Geometry: final body of the model. Coordinates: model frame, mm. A direction names the side the tool comes from. Round coordinates to 2 decimals unless told otherwise and drop trailing zeros. Write each loop counter-clockwise with the first axis right and the second up, starting at its lowest first coordinate (ties: lowest second). Pieces come first, ordered by that corner, then holes.
from build123d import *

# Parameters (mm, degrees)
SKETCH1_W               = 304.8
SKETCH1_H               = 171.45
BOSS_EXTRUDE1_DEPTH     = 19.05
SKETCH2_W               = 19.05
SKETCH2_H               = 19.05
BOSS_EXTRUDE2_DEPTH     = 19.05
SKETCH3_W               = 19.05
SKETCH3_H               = 19.05
CUT_EXTRUDE1_DEPTH      = 367.928913415
CUT_EXTRUDE2_DEPTH      = 367.928913415
CUT_EXTRUDE2_DEPTH_BACK = 367.928913415
CUT_EXTRUDE3_DEPTH      = 367.928913415
CUT_EXTRUDE3_DEPTH_BACK = 367.928913415
CUT_EXTRUDE4_DEPTH      = 367.928913415
SKETCH9_W               = 241.3
SKETCH9_H               = 171.45
BOSS_EXTRUDE3_DEPTH     = 19.05


with BuildPart() as part:
    # Sketch1 → Boss-Extrude1 (new body)
    with BuildSketch(Plane(origin=(0, 0, 0), x_dir=(1, 0, 0), z_dir=(0, 1, 0))):
        with Locations((-152.4, 85.725)):
            Rectangle(SKETCH1_W, SKETCH1_H)
    extrude(amount=BOSS_EXTRUDE1_DEPTH)

    # Mirror1: part across plane


with BuildPart() as part_1:
    add(part.part)
    add(part.part.mirror(Plane(origin=(0, 19.05, 0), x_dir=(0, 0, 1), z_dir=(-1, 0, 0))))

    # Sketch2 → Boss-Extrude2 (add)
    with BuildSketch(Plane(origin=(0, 19.05, 0), x_dir=(1, 0, 0), z_dir=(0, 1, 0))):
        with Locations((-314.325, 28.575)):
            Rectangle(SKETCH2_W, SKETCH2_H)
        with Locations((-314.325, 104.775)):
            Rectangle(SKETCH2_W, SKETCH2_H)
        with Locations((314.325, 142.875)):
            Rectangle(SKETCH2_W, SKETCH2_H)
        with Locations((314.325, 66.675)):
            Rectangle(SKETCH2_W, SKETCH2_H)
    extrude(amount=-BOSS_EXTRUDE2_DEPTH)

    # Sketch3 → Cut-Extrude1 (cut, symmetric)
    with BuildSketch(Plane(origin=(0, 19.05, 0), x_dir=(1, 0, 0), z_dir=(0, 1, 0))):
        with Locations((-104.775, 9.525)):
            Rectangle(SKETCH3_W, SKETCH3_H)
        with Locations((-104.775, 161.925)):
            Rectangle(SKETCH3_W, SKETCH3_H)
    cut_extrude1 = extrude(amount=CUT_EXTRUDE1_DEPTH, both=True, mode=Mode.SUBTRACT)

    # Mirror2: Cut-Extrude1 across plane
    add(cut_extrude1.mirror(Plane(origin=(0, 0, 0), x_dir=(0, 0, 1), z_dir=(1, 0, 0))), mode=Mode.SUBTRACT)

    # Sketch5 → Cut-Extrude2 (cut, two sides: drawn at the far end of the back side and taken through both)
    with BuildSketch(Plane(origin=(0, 19.05, 0), x_dir=(1, 0, 0), z_dir=(0, 1, 0)).offset(-CUT_EXTRUDE2_DEPTH_BACK)):
        with BuildLine():
            Line((9.525, 131.490128061), (9.525, 141.559871939))
            ThreePointArc((9.525, 141.559871939), (9.525, 146.05), (5.034871939, 146.05))
            Line((5.034871939, 146.05), (-5.034871939, 146.05))
            ThreePointArc((-5.034871939, 146.05), (-9.525, 146.05), (-9.525, 141.559871939))
            Line((-9.525, 141.559871939), (-9.525, 131.490128061))
            ThreePointArc((-9.525, 131.490128061), (-9.525, 127), (-5.034871939, 127))
            Line((-5.034871939, 127), (5.034871939, 127))
            ThreePointArc((5.034871939, 127), (9.525, 127), (9.525, 131.490128061))
        make_face()
        with BuildLine():
            Line((9.525, 80.690128061), (9.525, 90.759871939))
            ThreePointArc((9.525, 90.759871939), (9.525, 95.25), (5.034871939, 95.25))
            Line((5.034871939, 95.25), (-5.034871939, 95.25))
            ThreePointArc((-5.034871939, 95.25), (-9.525, 95.25), (-9.525, 90.759871939))
            Line((-9.525, 90.759871939), (-9.525, 80.690128061))
            ThreePointArc((-9.525, 80.690128061), (-9.525, 76.2), (-5.034871939, 76.2))
            Line((-5.034871939, 76.2), (5.034871939, 76.2))
            ThreePointArc((5.034871939, 76.2), (9.525, 76.2), (9.525, 80.690128061))
        make_face()
        with BuildLine():
            Line((9.525, 29.890128061), (9.525, 39.959871939))
            ThreePointArc((9.525, 39.959871939), (9.525, 44.45), (5.034871939, 44.45))
            Line((5.034871939, 44.45), (-5.034871939, 44.45))
            ThreePointArc((-5.034871939, 44.45), (-9.525, 44.45), (-9.525, 39.959871939))
            Line((-9.525, 39.959871939), (-9.525, 29.890128061))
            ThreePointArc((-9.525, 29.890128061), (-9.525, 25.4), (-5.034871939, 25.4))
            Line((-5.034871939, 25.4), (5.034871939, 25.4))
            ThreePointArc((5.034871939, 25.4), (9.525, 25.4), (9.525, 29.890128061))
        make_face()
    extrude(amount=CUT_EXTRUDE2_DEPTH + CUT_EXTRUDE2_DEPTH_BACK, mode=Mode.SUBTRACT)

    # Sketch6 → Cut-Extrude3 (cut, two sides: drawn at the far end of the back side and taken through both)
    with BuildSketch(Plane(origin=(0, 19.05, 0), x_dir=(1, 0, 0), z_dir=(0, 1, 0)).offset(-CUT_EXTRUDE3_DEPTH_BACK)):
        with BuildLine():
            Line((-114.3, 166.959871939), (-114.3, 156.890128061))
            ThreePointArc((-114.3, 156.890128061), (-114.3, 152.4), (-109.809871939, 152.4))
            Line((-109.809871939, 152.4), (-99.740128061, 152.4))
            ThreePointArc((-99.740128061, 152.4), (-95.25, 152.4), (-95.25, 156.890128061))
            Line((-95.25, 156.890128061), (-95.25, 166.959871939))
            Line((-95.25, 166.959871939), (-114.3, 166.959871939))
        make_face()
        with BuildLine():
            ThreePointArc((114.3, 156.890128061), (114.3, 152.4), (109.809871939, 152.4))
            Line((109.809871939, 152.4), (99.740128061, 152.4))
            ThreePointArc((99.740128061, 152.4), (95.25, 152.4), (95.25, 156.890128061))
            Line((95.25, 156.890128061), (95.25, 166.959871939))
            Line((95.25, 166.959871939), (114.3, 166.959871939))
            Line((114.3, 166.959871939), (114.3, 156.890128061))
        make_face()
        with BuildLine():
            ThreePointArc((95.25, 14.559871939), (95.25, 19.05), (99.740128061, 19.05))
            Line((99.740128061, 19.05), (109.809871939, 19.05))
            ThreePointArc((109.809871939, 19.05), (114.3, 19.05), (114.3, 14.559871939))
            Line((114.3, 14.559871939), (114.3, 4.490128061))
            Line((114.3, 4.490128061), (95.25, 4.490128061))
            Line((95.25, 4.490128061), (95.25, 14.559871939))
        make_face()
        with BuildLine():
            Line((-95.25, 4.490128061), (-95.25, 14.559871939))
            ThreePointArc((-95.25, 14.559871939), (-95.25, 19.05), (-99.740128061, 19.05))
            Line((-99.740128061, 19.05), (-109.809871939, 19.05))
            ThreePointArc((-109.809871939, 19.05), (-114.3, 19.05), (-114.3, 14.559871939))
            Line((-114.3, 14.559871939), (-114.3, 4.490128061))
            Line((-114.3, 4.490128061), (-95.25, 4.490128061))
        make_face()
    extrude(amount=CUT_EXTRUDE3_DEPTH + CUT_EXTRUDE3_DEPTH_BACK, mode=Mode.SUBTRACT)

    # Sketch8 → Cut-Extrude4 (cut, through all)
    with BuildSketch(Plane(origin=(0, 19.05, 0), x_dir=(1, 0, 0), z_dir=(0, 1, 0))):
        with BuildLine():
            Line((-304.8, 120.65), (-304.8, 114.3))
            ThreePointArc((-304.8, 114.3), (-301.625, 117.475), (-304.8, 120.65))
        make_face()
        with BuildLine():
            Line((-304.8, 95.25), (-304.8, 88.9))
            ThreePointArc((-304.8, 88.9), (-301.625, 92.075), (-304.8, 95.25))
        make_face()
        with BuildLine():
            Line((-304.8, 44.45), (-304.8, 38.1))
            ThreePointArc((-304.8, 38.1), (-301.625, 41.275), (-304.8, 44.45))
        make_face()
        with BuildLine():
            Line((-304.8, 19.05), (-304.8, 12.7))
            ThreePointArc((-304.8, 12.7), (-301.625, 15.875), (-304.8, 19.05))
        make_face()
        with BuildLine():
            ThreePointArc((304.8, 158.75), (301.625, 155.575), (304.8, 152.4))
            Line((304.8, 152.4), (304.8, 158.75))
        make_face()
        with BuildLine():
            ThreePointArc((304.8, 133.35), (301.625, 130.175), (304.8, 127))
            Line((304.8, 127), (304.8, 133.35))
        make_face()
        with BuildLine():
            ThreePointArc((304.8, 57.15), (301.625, 53.975), (304.8, 50.8))
            Line((304.8, 50.8), (304.8, 57.15))
        make_face()
        with BuildLine():
            ThreePointArc((304.8, 82.55), (301.625, 79.375), (304.8, 76.2))
            Line((304.8, 76.2), (304.8, 82.55))
        make_face()
    extrude(amount=-CUT_EXTRUDE4_DEPTH, mode=Mode.SUBTRACT)

    # Sketch9 → Boss-Extrude3 (add)
    with BuildSketch(Plane(origin=(0, 19.05, 0), x_dir=(1, 0, 0), z_dir=(0, 1, 0))):
        with Locations((0, 85.725)):
            Rectangle(SKETCH9_W, SKETCH9_H)
    extrude(amount=-BOSS_EXTRUDE3_DEPTH)


solid = part_1.part
1) Section A-A on y = 12. Output: boundary loops of the cut face in (x, z) (3 decimals), plus the area to 3 significant figures.
2) Line query: probe 1 along X at (y, z) = (13.75, -61); probe 2 along X at (y, z) = (15.25, -49). Output: solid intervals per line, ascending.
3) Section B-B on z = -69. Output: boundary loops of the cut face in (x, y), plus the area to 3 significant figures.
4) First-contact query: P1, Ø5.5, axis at x = -311.5, y = 6.5, coming from the -Z side; P2, Ø4, axis at x = 13.5, y = 8, coming from the +Z side; P3, Ø4, axis at y = 13.5, z = -3.5, coming from the -X side; P4, Ø9.5, axis at x = 312.5, y = 8.5, coming from the -Z side. Flat tips, straight axial feed; report the tip coordinate or a pass-through.
5) Reachability of faces 4 (the flat face through (-314, 10, -95.25)), 5 (the flat face through (-314, 10, -114.3)), 6 (the flat face through (314, 10, -152.4)), 7 (the flat face through (314, 10, -133.35)) from +Z, -Z, +X, -X, +Y, -Y: full face, straight path, thin tool, end or side. Return the list, or none.
6) Draft query along Z for faces 1 (the flat face through (-323.85, 10, -105)), 2 (the flat face through (314, 10, -57.15)), 3 (the flat face through (-304.8, 9, -66)). Return one class per face: pulls with the +Z half, pulls with the -Z half, needs draft (parallel to the pull), parting line crosses it, or undercut.
Filled in:
1. outline: (-323.85, -114.3) - (-304.8, -114.3) arc R3.175 cw to (-304.8, -120.65) - (-304.8, -171.45) - (304.8, -171.45) - (304.8, -158.75) arc R3.175 cw to (304.8, -152.4) - (323.85, -152.4) - (323.85, -133.35) - (304.8, -133.35) arc R3.175 cw to (304.8, -127) - (304.8, -82.55) arc R3.175 cw to (304.8, -76.2) - (323.85, -76.2) - (323.85, -57.15) - (304.8, -57.15) arc R3.175 cw to (304.8, -50.8) - (304.8, 0) - (-304.8, 0) - (-304.8, -12.7) arc R3.175 cw to (-304.8, -19.05) - (-323.85, -19.05) - (-323.85, -38.1) - (-304.8, -38.1) arc R3.175 cw to (-304.8, -44.45) - (-304.8, -88.9) arc R3.175 cw to (-304.8, -95.25) - (-323.85, -95.25) - close
1. area: 106,000 mm2
2. probe 1: x = -304.8 to 323.85
2. probe 2: x = -304.8 to 304.8
3. outline: (-304.8, 0) - (323.85, 0) - (323.85, 19.05) - (-304.8, 19.05) - close
3. area: 12,000 mm2
4. P1: stops at z = -114.3
4. P2: stops at z = 0
4. P3: stops at x = -304.8
4. P4: stops at z = -152.4
5. face 4: -X, +Y, -Y
5. face 5: -Z, -X, +Y, -Y
5. face 6: -Z, +X, +Y, -Y
5. face 7: +X, +Y, -Y
6. face 1: needs draft
6. face 2: pulls with the +Z half
6. face 3: undercut
